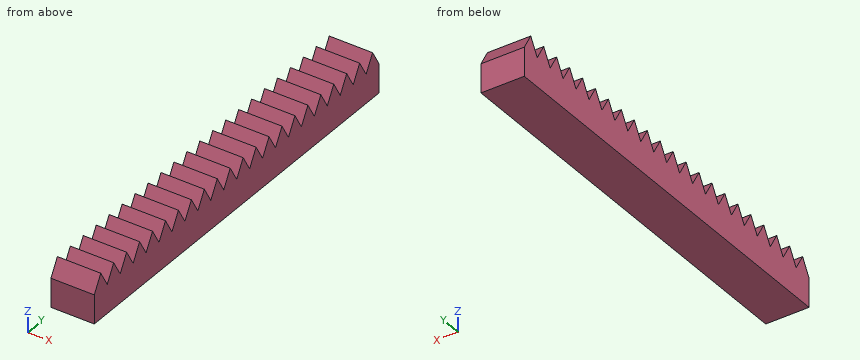
from build123d import *

# Parameters (mm, degrees)
F1_DEPTH = 3.75


with BuildPart() as f1:
    # F0 (on Right) → F1 (new body, symmetric)
    with BuildSketch(Plane.YZ):
        Polygon((35.795455, -2.5), (35.795455, 2.5), (32.541322, 2.5), (29.28719, 2.5), (26.033058, 2.5), (22.778926, 2.5), (19.524793, 2.5), (16.270661, 2.5), (13.016529, 2.5), (9.762397, 2.5), (6.508264, 2.5), (3.254132, 2.5), (0, 2.5), (-3.254132, 2.5), (-6.508264, 2.5), (-9.762397, 2.5), (-13.016529, 2.5), (-16.270661, 2.5), (-19.524793, 2.5), (-22.778926, 2.5), (-26.033058, 2.5), (-29.28719, 2.5), (-32.541322, 2.5), (-35.795455, 2.5), (-35.795455, -2.5), align=None)
        Polygon((26.033058, 2.5), (29.28719, 2.5), (27.660124, 5.318161), align=None)
        Polygon((29.28719, 2.5), (32.541322, 2.5), (30.914256, 5.318161), align=None)
        Polygon((32.541322, 2.5), (35.795455, 2.5), (34.168388, 5.318161), align=None)
        Polygon((13.016529, 2.5), (16.270661, 2.5), (14.643595, 5.318161), align=None)
        Polygon((6.508264, 2.5), (9.762397, 2.5), (8.135331, 5.318161), align=None)
        Polygon((16.270661, 2.5), (19.524793, 2.5), (17.897727, 5.318161), align=None)
        Polygon((9.762397, 2.5), (13.016529, 2.5), (11.389463, 5.318161), align=None)
        Polygon((-34.168388, 5.318161), (-35.795455, 2.5), (-32.541322, 2.5), align=None)
        Polygon((-30.914256, 5.318161), (-32.541322, 2.5), (-29.28719, 2.5), align=None)
        Polygon((-27.660124, 5.318161), (-29.28719, 2.5), (-26.033058, 2.5), align=None)
        Polygon((-24.405992, 5.318161), (-26.033058, 2.5), (-22.778926, 2.5), align=None)
        Polygon((-21.15186, 5.318161), (-22.778926, 2.5), (-19.524793, 2.5), align=None)
        Polygon((-17.897727, 5.318161), (-19.524793, 2.5), (-16.270661, 2.5), align=None)
        Polygon((-14.643595, 5.318161), (-16.270661, 2.5), (-13.016529, 2.5), align=None)
        Polygon((-11.389463, 5.318161), (-13.016529, 2.5), (-9.762397, 2.5), align=None)
        Polygon((-8.135331, 5.318161), (-9.762397, 2.5), (-6.508264, 2.5), align=None)
        Polygon((-6.508264, 2.5), (-3.254132, 2.5), (-4.881198, 5.318161), align=None)
        Polygon((-3.254132, 2.5), (0, 2.5), (-1.627066, 5.318161), align=None)
        Polygon((0, 2.5), (3.254132, 2.5), (1.627066, 5.318161), align=None)
        Polygon((3.254132, 2.5), (6.508264, 2.5), (4.881198, 5.318161), align=None)
        Polygon((19.524793, 2.5), (22.778926, 2.5), (21.15186, 5.318161), align=None)
        Polygon((22.778926, 2.5), (26.033058, 2.5), (24.405992, 5.318161), align=None)
    extrude(amount=F1_DEPTH, both=True)


solid = f1.part
Build history of the part. All positions in model axes, mm. Give positions to 0.01 mm unless a question says otherwise; leave off trailing zeros. Write each loop counter-clockwise with the first axis right and the second up, starting at its lowest first coordinate (ties: lowest second). Pieces come first, ordered by that corner, then holes. Notation, with made-up numbers: (83.25, 11.5) - (122.25, 11.5) arc R18 ccw to (122.25, 31.5) - close; hole circle Ø5 at (26, 46). An arc over 180 degrees is marked (long way). Use one line per item in the form item = value. Start each with the question number.
1. Band-saw the part on B-B on y = 17. Write the cut outline in (x, z).
2. Probe line 1 (Z direction, x = 3.25, y = -26); line 2 (Z direction, x = -2.5, y = -13.5). List the from-to ranges inside material, lowest first. Write a range as [from, to].
3. Band-saw the part on A-A on z = 4.5. Count the separate pieces of the cut face and the enclosed holes in it, plus the area to 3 significant figures.
4. Band-saw the part on C-C on y = -4. Write the cut outline in (x, z).
Conclusion:
q1.outline = (-3.75, -2.5) - (3.75, -2.5) - (3.75, 3.76) - (-3.75, 3.76) - close
q2.line_1 = [-2.5, 2.56]
q2.line_2 = [-2.5, 3.34]
q3.separate_pieces = 22
q3.enclosed_holes = 0
q3.area = 156 mm²
q4.outline = (-3.75, -2.5) - (3.75, -2.5) - (3.75, 3.79) - (-3.75, 3.79) - close
